For this review, take the finished solid that the model builds, in its own axes (mm). A direction names the side the tool comes from. Give positions to 0.01 mm unless a question says otherwise; leave off trailing zeros. Write each loop counter-clockwise with the first axis right and the second up, starting at its lowest first coordinate (ties: lowest second). Pieces come first, ordered by that corner, then holes. Notation, with made-up numbers: M 61.5,-25 L 86.5,-25 A21 cw 86.5,-5 Z; hole C 47,15.25 d9. An arc over 180 degrees is marked long. Use one line per item in the form item = value. Start each with the question number.
Q1. For probe 1 along Y at (x, z) = (0, -7.75); probe 2 along X at (y, z) = (-5, -0.25); probe 3 along Y at (x, z) = (-3.5, -5), list the stretches that pass through material, from the lowest coordinate up. Write a range as [from, to].
Q2. Clearance check with a flat-ended pin moving along its axis: pin 1 Ø20 at (x, y) = (0, 0) entering from -Z. State where the tip first meets the part, or that it passes through.
Q3. Consider section D-D on y = 18.5. Write out the cut boundary in (x, z).
Q4. Consider section B-B on x = 0. Write out the cut boundary in (y, z).
Q5. Consider section C-C on z = -2.75. Write out the cut boundary in (x, y).
Q6. Tool access review of faces 1 (the flat face through (-2, 12, -9.144)), 2 (the flat face through (30.824, 1, -4)): name each direction out of +Z, -Z, +X, -X, +Y, -Y from which nothing blocks a thin tool from reaching the whole face with its end or side.
Q7. Consider section A-A on y = 0. Write out the cut boundary in (x, z).
```python
from build123d import *

# Parameters (mm, degrees)
F1_DEPTH = 9.144
F2_W     = 64.972662
F2_H     = 38.302661
F3_DEPTH = 7.366
F5_D     = 12.5


with BuildPart() as f1:
    # F0 (on Top) → F1 (new body)
    with BuildSketch(Plane.XY):
        Polygon((49.50973, 36.174733), (0, 36.174733), (-52.063245, 36.174733), (-52.063245, -27.095586), (49.50973, -27.095586), align=None)
    extrude(amount=-F1_DEPTH)

    # F2 (on Top) → F3 (cut)
    with BuildSketch(Plane.XY):
        with Locations((-1.661934, 1.418617)):
            Rectangle(F2_W, F2_H)
    extrude(amount=-F3_DEPTH, mode=Mode.SUBTRACT)

    # F5 (through all)
    with Locations(Plane.XY):
        with Locations((0, 0)):
            Hole(F5_D / 2)


solid = f1.part
```
Working result:
q1.probe_1 = [-27.1, -6.25], [6.25, 36.17]
q1.probe_2 = [-52.06, -34.15], [30.82, 49.51]
q1.probe_3 = [-27.1, -17.73], [20.57, 36.17]
q2.pin_1 = -9.14
q3.outline = M -52.06,-9.14 L 49.51,-9.14 L 49.51,0 L 30.82,0 L 30.82,-7.37 L -34.15,-7.37 L -34.15,0 L -52.06,0 Z
q4.outline = M -27.1,-9.14 L -6.25,-9.14 L -6.25,-7.37 L -17.73,-7.37 L -17.73,0 L -27.1,0 Z; M 6.25,-9.14 L 36.17,-9.14 L 36.17,0 L 20.57,0 L 20.57,-7.37 L 6.25,-7.37 Z
q5.outline = M -52.06,-27.1 L 49.51,-27.1 L 49.51,36.17 L -52.06,36.17 Z; hole M -34.15,-17.73 L 30.82,-17.73 L 30.82,20.57 L -34.15,20.57 Z
q6.face_1 = -Z, +X, -X, +Y, -Y
q6.face_2 = +Z
q7.outline = M -52.06,-9.14 L -6.25,-9.14 L -6.25,-7.37 L -34.15,-7.37 L -34.15,0 L -52.06,0 Z; M 6.25,-9.14 L 49.51,-9.14 L 49.51,0 L 30.82,0 L 30.82,-7.37 L 6.25,-7.37 Z
